CAD build for the part. Positions are in the model's coordinates, mm. Face numbers are marked on the shaded views. A direction names the side the tool comes from. Coordinates: 2 decimals unless noted, no trailing zeros. Write each loop counter-clockwise with the first axis right and the second up, starting at its lowest first coordinate (ties: lowest second). Pieces come first, ordered by that corner, then holes. Notation, with made-up numbers: (69, 2) - (112, 2) arc R20 ccw to (112, 21) - close; hole circle Ø8 at (6.5, 14). An arc over 180 degrees is marked (long way). One line per question, with ' | ' between items. Start each with the question number.
1. Which spindle directions (+Z, -Z, +X, -X, +Y, -Y) get a long thin tool onto all of the face, cutting with end or side? Do the marked faces 1, 2, 3 and 4. Say none if no direction does.
2. Probe line 1 (X direction, y = -1780, z = 195.5); line 2 (Y direction, x = 156.5, z = 144); line 3 (Z direction, x = 600, y = -1608). List the from-to ranges inside material, lowest first.
3. Band-saw the part on C-C, the plane z = -361. Write the cut outline in (x, y), then the cut area to 3 significant figures.
4. Band-saw the part on D-D, the plane z = -158. Write the cut outline in (x, y).
5. Band-saw the part on B-B, the plane y = -927. Write the cut outline in (x, z).
6. Flat gauge pins, fed straight in: P1, Ø4.5, axis at x = 522, y = -1530.5, coming from the +Z side; P2, Ø6, axis at x = 702, z = -312, coming from the -Y side. Where does each tip first touch, or does it go through?
7. Band-saw the part on A-A, the plane x = 199.5. Write the cut outline in (y, z).
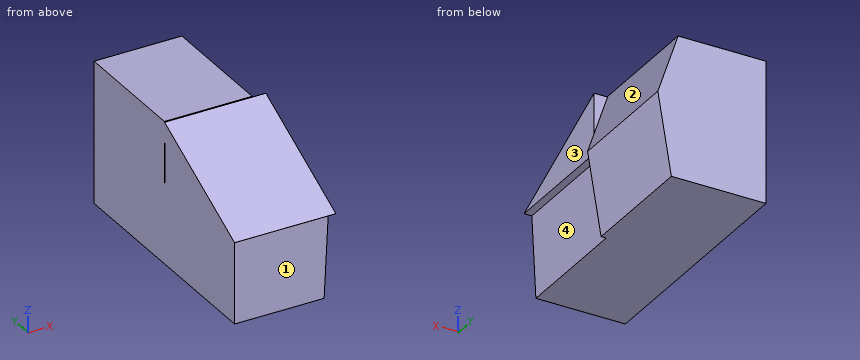
from build123d import *

# Parameters (mm, degrees)
F12_DEPTH = 914.4
F13_DEPTH = 914.4
F14_DEPTH = 762
F15_DEPTH = 914.4


with BuildPart() as f12:
    # F8 (on offset) → F12 (new body, through all)
    with BuildSketch(Plane.XZ.offset(2438.4)):
        Polygon((673.1, -609.6), (703.58, 0), (0, 0), (0, -609.6), align=None)
    extrude(amount=-F12_DEPTH)

    # F10 (on offset) → F13 (join, through all)
    with BuildSketch(Plane.XZ.offset(1524)):
        Polygon((0, 457.2), (0, 0), (673.1, 0), (584.2, 457.2), align=None)
        Polygon((673.1, 0), (0, 0), (0, -609.6), (609.6, -609.6), align=None)
    extrude(amount=-F13_DEPTH)

    # F11 (on Right) → F14 (join)
    with BuildSketch(Plane.YZ):
        Polygon((-1526.670575, 452.586561), (-2437.97636, 0), (-1533.226132, 0), align=None)
    extrude(amount=F14_DEPTH)

    # F9 (on offset) → F15 (join)
    with BuildSketch(Plane.XZ.offset(609.6)):
        Polygon((0, 457.2), (0, 0), (812.8, 0), (660.4, 457.2), align=None)
        Polygon((812.8, 0), (0, 0), (0, -609.6), (711.2, -609.6), align=None)
    extrude(amount=F15_DEPTH)


solid = f12.part
Filled in:
1) face 1: +Z, -Z, +X, -X, -Y | face 2: +Z, +X, +Y | face 3: +Z, -Z, +X, -Y | face 4: -Z, +X, -Y
2) line 1: x = 0 to 762 | line 2: y = -2148.03 to -1531.14, -1524 to -609.6 | line 3: z = -609.6 to 412.2
3) outline: (0, -2438.4) - (685.53, -2438.4) - (685.53, -1524) - (752.63, -1524) - (752.63, -609.6) - (0, -609.6) - close | area: 1,320,000 mm²
4) outline: (0, -2438.4) - (695.68, -2438.4) - (695.68, -1524) - (786.47, -1524) - (786.47, -609.6) - (0, -609.6) - close
5) outline: (0, -609.6) - (711.2, -609.6) - (812.8, 0) - (660.4, 457.2) - (0, 457.2) - close
6) P1: stops at z = 451.8 | P2: stops at y = -1524
7) outline: (-2438.4, -609.6) - (-609.6, -609.6) - (-609.6, 457.2) - (-1524, 457.2) - (-1524, 0) - (-1533.23, 0) - (-1526.67, 452.59) - (-2437.98, 0) - (-2438.4, 0) - close
